from build123d import *

# Parameters (mm, degrees)
SEMICIRCULAR_CAMERA_PLATFORM_DEPTH = 12


with BuildPart() as part:
    # 草图1 → Semicircular_camera_platform (new body)
    with BuildSketch(Plane.XY):
        Polygon((90, 0), (89.230037524, 11.7473573), (86.933324366, 23.293714059), (83.149157926, 34.441508913), (77.942286341, 45), (71.401800626, 54.788528611), (63.639610307, 63.639610307), (54.788528611, 71.401800626), (45, 77.942286341), (34.441508913, 83.149157926), (23.293714059, 86.933324366), (11.7473573, 89.230037524), (0, 90), (-11.7473573, 89.230037524), (-23.293714059, 86.933324366), (-34.441508913, 83.149157926), (-45, 77.942286341), (-54.788528611, 71.401800626), (-63.639610307, 63.639610307), (-71.401800626, 54.788528611), (-77.942286341, 45), (-83.149157926, 34.441508913), (-86.933324366, 23.293714059), (-89.230037524, 11.7473573), (-90, 0), align=None)
    extrude(amount=SEMICIRCULAR_CAMERA_PLATFORM_DEPTH)


solid = part.part
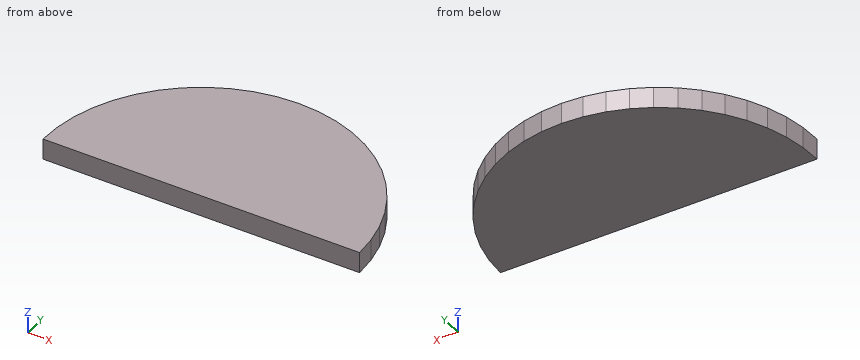
Build history of the part. All positions in model axes, mm. Give positions to 0.01 mm unless a question says otherwise; leave off trailing zeros. Order: outer loops, then holes, each group sorted by start corner. A loop starts at its lowest first (then second) coordinate and runs counter-clockwise, first axis right, second up. Notation, with made-up numbers: M -26,9 L -6,9 A7 cw -6,20 Z; hole C -12.5,37 d1. An arc over 180 degrees is marked long. Use one line per item in the form item = value.
1) Probe probe 1 along X at (y, z) = (34.5, 8.5); probe 2 along X at (y, z) = (12, 10.25); probe 3 along Y at (x, z) = (-61, 9.75). List the from-to ranges inside material, lowest first.
Calculated:
probe_1 = -83.12 to 83.12
probe_2 = -89.18 to 89.18
probe_3 = 0 to 65.95
2) Saw through at A-A (z = 5.75). Give the cut face in (x, y).
Calculated:
outline = M -90,0 L 90,0 L 89.23,11.75 L 86.93,23.29 L 83.15,34.44 L 77.94,45 L 71.4,54.79 L 63.64,63.64 L 54.79,71.4 L 45,77.94 L 34.44,83.15 L 23.29,86.93 L 11.75,89.23 L 0,90 L -11.75,89.23 L -23.29,86.93 L -34.44,83.15 L -45,77.94 L -54.79,71.4 L -63.64,63.64 L -71.4,54.79 L -77.94,45 L -83.15,34.44 L -86.93,23.29 L -89.23,11.75 Z
3) Drop flat-ended pins along their axis: pin 1 (2 mm diameter, centred on y = 38.5, z = 9, fed in from -X); pin 2 (4 mm diameter, centred on y = 40, z = 9.5, fed in from +X); pin 3 (1.5 mm diameter, centred on y = 76.5, z = 10.5, fed in from -X). Give the stop position or say it passes through.
Calculated:
pin_1 = -81.64
pin_2 = 81.39
pin_3 = -48.28
4) Saw through at C-C (x = -56.5). Give the cut face in (y, z).
Calculated:
outline = M 0,0 L 69.9,0 L 69.9,12 L 0,12 Z
5) Saw through at B-B (y = 76). Give the cut face in (x, z), plus the area to 3 significant figures.
Calculated:
outline = M -47.91,0 L 47.91,0 L 47.91,12 L -47.91,12 Z
area = 1,150 mm2
